Autodesk Inventor part; units mm, degrees
ref_plane "YZ Plane" through (0, 0, 0) normal (1, 0, 0) x (0, 1, 0)
ref_plane "XZ Plane" through (0, 0, 0) normal (0, 1, 0) x (-1, 0, 0)
ref_plane "XY Plane" through (0, 0, 0) normal (0, 0, 1) x (1, 0, 0)
sketch "Boceto1" plane through (0, 30.6548, -58.1067) normal (1, 0, 0) x (0, 1, 0)
  arc A0 (-13.6856, -6.1404) -> (15, 0) centre (0, 0) ccw
  arc A1 (-13.6856, -6.1404) -> (14.8675, 1.989) centre (0, 0) ccw
  arc A2 (-13.6856, -6.1404) -> (15, 0) centre (0, 0) ccw
  circle A3 centre (0, 0) radius 5
  arc A4 (-14.8673, 1.9912) -> (14.8675, 1.989) centre (0, 0) ccw
  arc A5 (-2.5, 90) -> (2.5, 90) centre (0, 90) ccw
  arc A6 (2.5, 150) -> (-2.5, 150) centre (0, 150) ccw
  line L0 (2.5, 150) -> (2.5, 90)
  line L1 (-2.5, 150) -> (-2.5, 90)
  line L2 (15, 0) -> (4.989, 150.3322)
  line L3 (-15, 0) -> (-5, 150)
  arc A7 (4.989, 150.3322) -> (-5, 150) centre (0, 150) ccw
  point P0 (15, 0)
  point P1 (15, 0)
extrude "Extrusión1" add sketch "Boceto1" along normal blind 3 contours A4 L3 A7 L2 A0
properties part number "CorrederaPalanca"
For this review, take the finished solid that the model builds, in its own axes (mm). A direction names the side the tool comes from. Coordinates: 2 decimals unless noted, no trailing zeros. Loops run counter-clockwise (first coordinate to the right, second up) from the corner with the lowest first, then second, coordinate; pieces in that order, holes last. Notation, with made-up numbers: (38, 57.25) - (62, 57.25) arc R22 cw to (62, 65.25) - close; hole circle Ø2 at (-36.75, 54). An arc over 180 degrees is marked (long way). Return JSON: item names as keys, results as strings.
Item 1: For faces 4 (the flat face through (1, 33.155, 62)), 5 (the flat face through (3, 30, -6)), list the 3-axis set-ups (+Z, -Z, +X, -X, +Y, -Y) from which the entire face can be reached by the end or side of a thin tool; tool diameter is ignored.
Determined:
{"face 4": "+X, -X", "face 5": "+Z, -Z, +X, +Y, -Y"}
Item 2: For line 1 (Z direction, x = 2.3, y = 29); line 2 (Z direction, x = 2.3, y = 27); line 3 (Z direction, x = 1.65, y = 35), list the stretches that pass through material, from the lowest coordinate up.
Determined:
{"line 1": "z = -73.02 to -62.82, -53.39 to 30.02, 93.77 to 96.61", "line 2": "z = -72.65 to -61.52, -54.69 to 95.31", "line 3": "z = -72.46 to -60.58, -55.63 to 94.37"}
Item 3: Mouldability with a two-part tool opening along Y and no side actions: class faces 1 (the cylindrical face through (1.479, 30.381, 96.886)), 2 (the flat face through (1, 28.155, 62)), 3 (the flat face through (0, 30, -6)) as pulls with the +Y half, pulls with the -Y half, needs draft (parallel to the pull), parting line crosses it, or undercut.
Determined:
{"face 1": "parting line crosses it", "face 2": "undercut", "face 3": "needs draft"}
Item 4: Take a section at B-B (x = 1.55). Give the boundary of the cut face in (y, z), then the cut area to 3 significant figures.
Determined:
{"outline": "(15.65, -58.11) arc R15 ccw to (16.97, -64.25) arc R15 ccw to (45.65, -58.11) - (35.64, 92.23) arc R5 ccw to (25.65, 91.89) - close; hole circle Ø10 at (30.65, -58.11); hole (28.15, 31.89) arc R2.5 ccw to (33.15, 31.89) - (33.15, 91.89) arc R2.5 ccw to (28.15, 91.89) - close", "area": "3,000 mm2"}
Item 5: Insertion check: pin 1 (1.5 mm diameter, centred on x = 1, y = 24.5, fed in from -Z); pin 2 (1.5 mm diameter, centred on x = 1.5, z = 75, fed in from -Y); pin 3 (1.5 mm diameter, centred on x = 2, z = 60.5, fed in from +Y). Each pin has a flat end and moves straight along its axis. Give the tip position at first contact, or say it passes through.
Determined:
{"pin 1": "stops at z = -72.1", "pin 2": "stops at y = 24.48", "pin 3": "stops at y = 37.81"}
Item 6: Take a section at A-A (y = 31). Give the boundary of the cut face in (x, z), then the cut area to 3 significant figures.
Determined:
{"outline": "(0, -73.1) - (3, -73.1) - (3, -63.09) - (0, -63.09) - close; (0, -53.12) - (3, -53.12) - (3, 29.42) - (0, 29.42) - close; (0, 94.37) - (3, 94.37) - (3, 96.88) - (0, 96.88) - close", "area": "285 mm2"}
Item 7: Take a section at D-D (y = 38.5). Give the boundary of the cut face in (x, z).
Determined:
{"outline": "(0, -70.89) - (3, -70.89) - (3, 49.33) - (0, 49.33) - close"}
Item 8: Take a section at C-C (z = -7). Give the boundary of the cut face in (x, y), then the cut area to 3 significant figures.
Determined:
{"outline": "(0, 19.06) - (3, 19.06) - (3, 42.25) - (0, 42.25) - close", "area": "69.6 mm2"}
